```python
from build123d import *

# Parameters (mm, degrees)
SKETCH1_W           = 508
SKETCH1_H           = 381
BOSS_EXTRUDE1_DEPTH = 1.6002
SKETCH5_R           = 3.2639
CUT_EXTRUDE1_DEPTH  = 2.54
SKETCH7_R           = 3.2639
CUT_EXTRUDE3_DEPTH  = 2.54
SKETCH8_W           = 49.2125
SKETCH8_H           = 69.85
SKETCH8_H_2         = 19.05
CUT_EXTRUDE4_DEPTH  = 318.504032478
SKETCH9_R           = 16.764
CUT_EXTRUDE5_DEPTH  = 318.504032478


with BuildPart() as part:
    # Sketch1 → Boss-Extrude1 (new body)
    with BuildSketch(Plane(origin=(0, 0, 0), x_dir=(0, 0, -1), z_dir=(1, 0, 0))):
        Rectangle(SKETCH1_W, SKETCH1_H)
    extrude(amount=BOSS_EXTRUDE1_DEPTH)

    # Sketch5 → Cut-Extrude1 (cut)
    with BuildSketch(Plane(origin=(1.6002, 0, 0), x_dir=(0, 0, -1), z_dir=(1, 0, 0))):
        with Locations((-245.11, 152.4)):
            Circle(SKETCH5_R)
        with Locations((-245.11, 76.2)):
            Circle(SKETCH5_R)
        with Locations((-245.11, 0)):
            Circle(SKETCH5_R)
        with Locations((-245.11, -76.2)):
            Circle(SKETCH5_R)
        with Locations((-245.11, -152.4)):
            Circle(SKETCH5_R)
        with Locations((245.11, 152.4)):
            Circle(SKETCH5_R)
        with Locations((245.11, 76.2)):
            Circle(SKETCH5_R)
        with Locations((245.11, 0)):
            Circle(SKETCH5_R)
        with Locations((245.11, -76.2)):
            Circle(SKETCH5_R)
        with Locations((245.11, -152.4)):
            Circle(SKETCH5_R)
    extrude(amount=-CUT_EXTRUDE1_DEPTH, mode=Mode.SUBTRACT)

    # Sketch7 → Cut-Extrude3 (cut)
    with BuildSketch(Plane(origin=(1.6002, 0, 0), x_dir=(0, 0, -1), z_dir=(1, 0, 0))):
        with Locations((-217.5002, 178.689)):
            Circle(SKETCH7_R)
        with Locations((-109.5502, 178.689)):
            Circle(SKETCH7_R)
        with Locations((-1.6002, 178.689)):
            Circle(SKETCH7_R)
        with Locations((106.3498, 178.689)):
            Circle(SKETCH7_R)
        with Locations((214.2998, 178.689)):
            Circle(SKETCH7_R)
    extrude(amount=-CUT_EXTRUDE3_DEPTH, mode=Mode.SUBTRACT)

    # Sketch8 → Cut-Extrude4 (cut, through all)
    with BuildSketch(Plane(origin=(1.6002, 0, 0), x_dir=(0, 0, -1), z_dir=(1, 0, 0))):
        with Locations((-152.4, 57.404)):
            Rectangle(SKETCH8_W, SKETCH8_H)
        with Locations((152.4, 57.404)):
            Rectangle(SKETCH8_W, SKETCH8_H)
        with Locations((152.4, -9.271)):
            Rectangle(SKETCH8_W, SKETCH8_H_2)
        with Locations((-152.4, -9.271)):
            Rectangle(SKETCH8_W, SKETCH8_H_2)
    extrude(amount=-CUT_EXTRUDE4_DEPTH, mode=Mode.SUBTRACT)

    # Sketch9 → Cut-Extrude5 (cut, through all)
    with BuildSketch(Plane(origin=(1.6002, 0, 0), x_dir=(0, 0, -1), z_dir=(1, 0, 0))):
        with Locations((0, -110.871)):
            Circle(SKETCH9_R)
    extrude(amount=-CUT_EXTRUDE5_DEPTH, mode=Mode.SUBTRACT)


solid = part.part
```
Geometry: final body of the model. Coordinates: model frame, mm. Coordinates: 2 decimals unless noted, no trailing zeros. Order: outer loops, then holes, each group sorted by start corner. A loop starts at its lowest first (then second) coordinate and runs counter-clockwise, first axis right, second up. Notation, with made-up numbers: (60.25, 8) -> (68.25, 8) arc R22 cw to (68.25, 37) -> close; hole circle Ø10 at (-14.75, 86.25). An arc over 180 degrees is marked (long way). Answer in a Markdown table with one row per item.
Item 1: Contact query for a flat-ended pin moving along its axis: P1, Ø4, axis at y = 152.4, z = -245.11, coming from the -X side. Output: stop coordinate, or through.
Return value:
| item | result |
|---|---|
| P1 | passes through |
Item 2: Ray query, L1, parallel to Z at x = 1.1, y = 85.5; L2, parallel to Y at x = 0.9, z = 152; L3, parallel to Y at x = 0.75, z = -245.11. Return the intervals inside material, ascending.
Return value:
| item | result |
|---|---|
| L1 | z = -254 to -177.01, -127.79 to 127.79, 177.01 to 254 |
| L2 | y = -190.5 to -18.8, 0.25 to 22.48, 92.33 to 190.5 |
| L3 | y = -190.5 to -155.66, -149.14 to -79.46, -72.94 to -3.26, 3.26 to 72.94, 79.46 to 149.14, 155.66 to 190.5 |
Item 3: Section A-A on z = 137. Output: boundary loops of the cut face in (x, y).
Return value:
| item | result |
|---|---|
| outline | (0, -190.5) -> (1.6, -190.5) -> (1.6, -18.8) -> (0, -18.8) -> close; (0, 0.25) -> (1.6, 0.25) -> (1.6, 22.48) -> (0, 22.48) -> close; (0, 92.33) -> (1.6, 92.33) -> (1.6, 190.5) -> (0, 190.5) -> close |
Item 4: Draft query along Y for faces 1 (the flat face through (0, 3, 4)), 2 (the cylindrical face through (0.811, -127.236, 3.634)). Return one class per face: released by +Y, released by -Y, zero draft, split by the parting line, or undercut.
Return value:
| item | result |
|---|---|
| face 1 | zero draft |
| face 2 | undercut |
Item 5: Section B-B on x = 0.95. State how many separate pieces and enclosed holes the cut face has, plus the area to 3 significant figures.
Return value:
| item | result |
|---|---|
| separate pieces | 1 |
| enclosed holes | 20 |
| area | 183,000 mm² |
